Print and shaded views of the part. All mm, measured from the part's lowest x, y and z. A direction names the side the tool comes from. Round coordinates to 2 decimals unless told otherwise and drop trailing zeros. Order: outer loops, then holes, each group sorted by start corner. A loop starts at its lowest first (then second) coordinate and runs counter-clockwise, first axis right, second up. Notation, with made-up numbers: (4, 61.5) - (52, 61.5) arc R12 ccw to (52, 76.5) - close; hole circle Ø11 at (47.5, 60.25). An arc over 180 degrees is marked (long way). Return JSON: item names as keys, results as strings. Group by question number.
Item 1: Saw through at C-C on z = 0.4. List the corners of the cut face in (x, y) (1 decimal), and give its area (3 significant figures).
Item 2: Saw through at B-B on y = 28.47. List the corners of the cut face in (x, z).
Item 3: Tool access for the marked faces 4 and 5: list every direction of +Z, -Z, +X, -X, +Y, -Y with a clear straight run to the whole face (end or side of a thin tool).
Item 4: Two-plate mould, pull along Y, no slides. Class the marked faces 1, 2 and 3: released by +Y, released by -Y, zero draft, split by the parting line, or undercut.
Item 5: Drop flat-ended pins along their axis: pin 1 (8 mm diameter, centred on x = 15, y = 26, fed in from -Z); pin 2 (2.5 mm diameter, centred on x = 17.5, y = 6.53, fed in from -Z); pin 3 (0.6 mm diameter, centred on x = 12.5, z = 0.5, fed in from -Y). Give the stop position or say it passes through.
Item 6: Probe probe 1 along Y at (x, z) = (17.5, 1.4); probe 2 along Y at (x, z) = (17, 0.8); probe 3 along Y at (x, z) = (8.5, 1.9). List the from-to ranges inside material, lowest first.
Item 7: Saw through at A-A on x = 17.5. List the corners of the cut face in (y, z).
Item 8: Saw through at D-D on x = 10. List the corners of the cut face in (y, z), and give its area (3 significant figures).
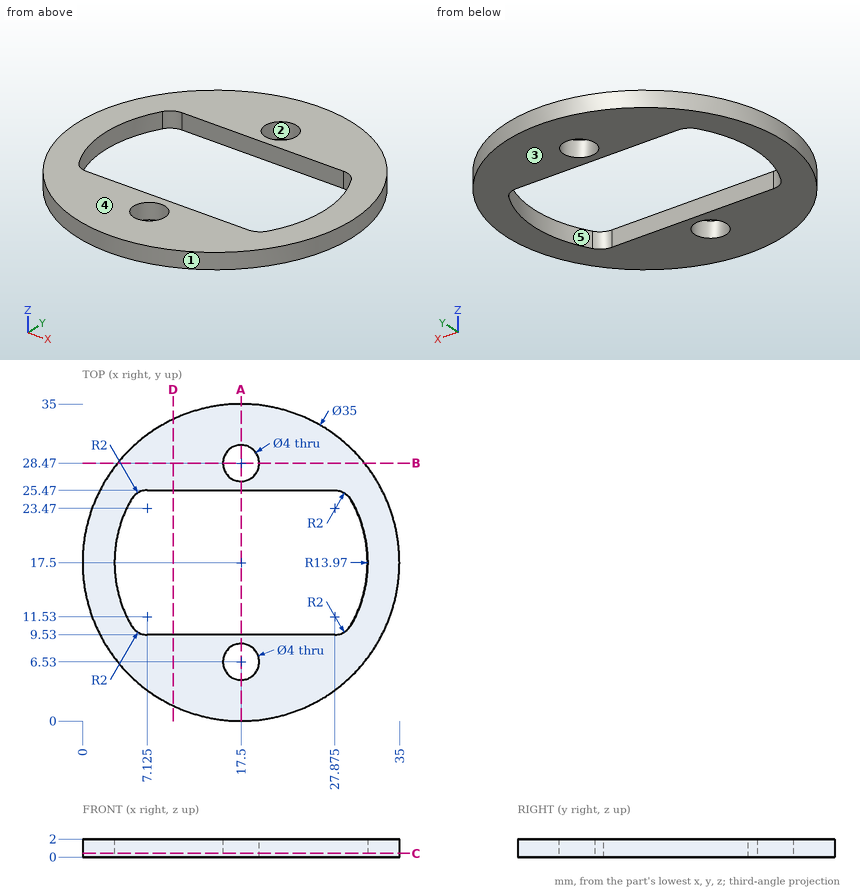
Filled in:
{
 "1": {"outline": "circle Ø35 at (17.5, 17.5); hole (5.4, 10.5) arc R2 ccw to (7.1, 9.5) - (27.9, 9.5) arc R2 ccw to (29.6, 10.5) arc R14 ccw to (29.6, 24.5) arc R2 ccw to (27.9, 25.5) - (7.1, 25.5) arc R2 ccw to (5.4, 24.5) arc R14 ccw to start; hole circle Ø4 at (17.5, 6.5); hole circle Ø4 at (17.5, 28.5)", "area": "518 mm^2"},
 "2": {"outline": "(3.87, 0) - (15.5, 0) - (15.5, 2) - (3.87, 2) - close; (19.5, 0) - (31.13, 0) - (31.13, 2) - (19.5, 2) - close"},
 "3": {"face 4": "+Z, +X, -X, +Y, -Y", "face 5": "+Z, -Z"},
 "4": {"face 1": "split by the parting line", "face 2": "undercut", "face 3": "zero draft"},
 "5": {"pin 1": "stops at z = 0", "pin 2": "passes through", "pin 3": "stops at y = 0.64"},
 "6": {"probe 1": "y = 0 to 4.53, 8.53 to 9.53, 25.47 to 26.47, 30.47 to 35", "probe 2": "y = 0.01 to 4.59, 8.47 to 9.53, 25.47 to 26.53, 30.41 to 34.99", "probe 3": "y = 2.49 to 9.53, 25.47 to 32.51"},
 "7": {"outline": "(0, 0) - (4.53, 0) - (4.53, 2) - (0, 2) - close; (8.53, 0) - (9.53, 0) - (9.53, 2) - (8.53, 2) - close; (25.47, 0) - (26.47, 0) - (26.47, 2) - (25.47, 2) - close; (30.47, 0) - (35, 0) - (35, 2) - (30.47, 2) - close"},
 "8": {"outline": "(1.69, 0) - (9.53, 0) - (9.53, 2) - (1.69, 2) - close; (25.47, 0) - (33.31, 0) - (33.31, 2) - (25.47, 2) - close", "area": "31.4 mm^2"}
}
